```python
from build123d import *

# Parameters (mm, degrees)
CUT_EXTRUDE1_DEPTH = 3.175
FILLET1_R          = 0.79375
CHAMFER1_SIZE      = 0.254
CHAMFER2_SIZE      = 0.762


with BuildPart() as part:
    # Sketch1 → Revolve1 (revolve)
    with BuildSketch(Plane.XY):
        Polygon((3.175, 0), (6.35, 0), (6.35, 6.35), (2.9845, 6.35), (2.9845, 47.625), (1.5875, 47.625), (1.5875, 3.175), (3.175, 3.175), align=None)
    revolve(axis=Axis((0, 5.569325848, 0), (0, -1, 0)))

    # Sketch2 → Cut-Extrude1 (cut)
    with BuildSketch(Plane.XZ):
        Polygon((1.833087105, 3.175), (-1.833087105, 3.175), (-3.666174209, 0), (-1.833087105, -3.175), (1.833087105, -3.175), (3.666174209, 0), align=None)
    extrude(amount=-CUT_EXTRUDE1_DEPTH, mode=Mode.SUBTRACT)

    # Fillet1
    fillet1_edges = [part.edges().sort_by_distance(p)[0] for p in [
        (0, 3.175, 3.175),
        (-2.749630657, 3.175, 1.5875),
        (-2.749630657, 3.175, -1.5875),
        (0, 3.175, -3.175),
        (2.749630657, 3.175, -1.5875),
        (2.749630657, 3.175, 1.5875),
        (-1.833087105, 1.5875, 3.175),
        (-3.666174209, 1.5875, 0),
        (-1.833087105, 1.5875, -3.175),
        (1.833087105, 1.5875, -3.175),
        (3.666174209, 1.5875, 0),
        (1.833087105, 1.5875, 3.175),
        (-2.9845, 6.35, 0),
    ]]
    fillet(fillet1_edges, radius=FILLET1_R)

    # Chamfer1
    chamfer1_edges = [part.edges().sort_by_distance(p)[0] for p in [
        (-1.5875, 3.175, 0),
        (0, 0, 3.175),
        (2.749630657, 0, 1.5875),
        (-1.5875, 47.625, 0),
        (2.749630657, 0, -1.5875),
        (0, 0, -3.175),
        (-2.9845, 47.625, 0),
        (-2.749630657, 0, -1.5875),
        (-2.749630657, 0, 1.5875),
        (-1.771690329, 0, 3.068657664),
        (1.771690329, 0, 3.068657664),
        (3.543380657, 0, 0),
        (1.771690329, 0, -3.068657664),
        (-1.771690329, 0, -3.068657664),
        (-3.543380657, 0, 0),
    ]]
    chamfer(chamfer1_edges, length=CHAMFER1_SIZE)

    # Chamfer2
    chamfer2_edges = [part.edges().sort_by_distance(p)[0] for p in [
        (-6.35, 6.35, 0),
        (-6.35, 0, 0),
    ]]
    chamfer(chamfer2_edges, length=CHAMFER2_SIZE)


solid = part.part
```
Can you work these out from the model? Positions are in its coordinate system, mm. Coordinates: 2 decimals unless noted, no trailing zeros. Loops run counter-clockwise (first coordinate to the right, second up) from the corner with the lowest first, then second, coordinate; pieces in that order, holes last. Notation, with made-up numbers: (-11, 71.5) -> (-5, 71.5) arc R32 cw to (-5, 109.5) -> close; hole circle Ø5 at (16.5, 67). An arc over 180 degrees is marked (long way). Answer as a JSON object with one key per item and string values.
1) For P1, Ø3, axis at x = 0, z = 0, coming from the -Y side; P2, Ø1.5, axis at x = 0.5, y = 19.5, coming from the +Z side; P3, Ø4, axis at x = 4, z = 3.5, coming from the +Y side; P4, Ø5, axis at y = 31, z = 0.5, coming from the -X side, each with a flat end and sliding along its axis, tell me the tip position at first contact or that it passes through.
Results:
{"P1": "passes through", "P2": "stops at z = 2.98", "P3": "stops at y = 6.5", "P4": "stops at x = -2.98"}
2) Imagine slicing it at C-C (y = 42.5). Please give me the cut outline in (x, z) (1 decimal), then the cut area to 3 significant figures.
Results:
{"outline": "circle Ø6 at (0, 0); hole circle Ø3.2 at (0, 0)", "area": "20.1 mm^2"}
3) Thinking about a two-plate mould opening in X: for faces 1 (the face through (1, 6.35, -4)), 2 (the face through (-0.647, 27.539, -2.914)), 3 (the face through (-0.34, 25.09, -1.55)), which applies, pulls with the +X half, pulls with the -X half, needs draft (parallel to the pull), parting line crosses it, or undercut?
Results:
{"face 1": "needs draft", "face 2": "parting line crosses it", "face 3": "undercut"}
4) If I drill on line 1 (Z direction, x = 0, y = 38); line 2 (Y direction, x = 3.5, z = -1.5); line 3 (X direction, y = 11, z = -1.25), over which ranges is the centre line in solid material (lowest first)?
Results:
{"line 1": "z = -2.98 to -1.59, 1.59 to 2.98", "line 2": "y = 0 to 6.35", "line 3": "x = -2.71 to -0.98, 0.98 to 2.71"}
